Verification items for the finished model (mm, model axes). A direction names the side the tool comes from. Give positions to 0.01 mm unless a question says otherwise; leave off trailing zeros. Write each loop counter-clockwise with the first axis right and the second up, starting at its lowest first coordinate (ties: lowest second). Pieces come first, ordered by that corner, then holes. Notation, with made-up numbers: (12, -14) -> (59, -14) arc R5 cw to (59, -6) -> close; hole circle Ø5 at (62, -28). An arc over 180 degrees is marked (long way). Write item = value, one per line.
from build123d import *

# Parameters (mm, degrees)
BOSS_EXTRUDE1_DEPTH          = 2.286
SKETCH2_W                    = 25.4
SKETCH2_H                    = 2.286
BOSS_EXTRUDE2_DEPTH          = 20.828
F_10_0_1935_DIAMETER_HOLE1_D = 4.9149
F_10_0_1935_DIAMETER_HOLE2_D = 4.9149
F_10_0_1935_DIAMETER_HOLE3_D = 4.9149
CUT_EXTRUDE1_DEPTH           = 50.8
FILLET1_R                    = 2.54
FILLET2_R                    = 2.54


with BuildPart() as part:
    # Sketch1 → Boss-Extrude1 (new body)
    with BuildSketch(Plane(origin=(0, 0, 0), x_dir=(1, 0, 0), z_dir=(0, 1, 0))):
        Polygon((19.05, 34.925), (-19.05, 34.925), (-19.05, 4.22504843), (-63.051024839, 14.626449943), (-71.815919826, -22.451665109), (-19.05, -34.925), (19.05, -34.925), align=None)
    extrude(amount=BOSS_EXTRUDE1_DEPTH)

    # Sketch2 → Boss-Extrude2 (add)
    with BuildSketch(Plane(origin=(0, 2.286, 0), x_dir=(1, 0, 0), z_dir=(0, 1, 0))):
        with Locations((0, -33.782)):
            Rectangle(SKETCH2_W, SKETCH2_H)
    extrude(amount=BOSS_EXTRUDE2_DEPTH)

    # #10 (0.1935) Diameter Hole1 (through all)
    with Locations(Plane(origin=(0, 2.286, 0), x_dir=(1, 0, 0), z_dir=(0, 1, 0))):
        with Locations((-12.7, -24.735), (12.7, -24.735), (-12.7, 19.715), (12.7, 19.715)):
            Hole(F_10_0_1935_DIAMETER_HOLE1_D / 2)

    # #10 (0.1935) Diameter Hole2 (through all)
    with Locations(Plane(origin=(0, 0, 32.639), x_dir=(-1, 0, 0), z_dir=(0, 0, -1))):
        with Locations((0, 14.859)):
            Hole(F_10_0_1935_DIAMETER_HOLE2_D / 2)

    # #10 (0.1935) Diameter Hole3 (through all)
    with Locations(Plane(origin=(0, 2.286, 0), x_dir=(1, 0, 0), z_dir=(0, 1, 0))):
        with Locations((-48.685323349, 4.705533941), (-36.325951665, 1.783902278), (-54.528586674, -20.013209428), (-42.169214989, -22.93484109)):
            Hole(F_10_0_1935_DIAMETER_HOLE3_D / 2)

    # Sketch10 → Cut-Extrude1 (cut)
    with BuildSketch(Plane(origin=(0, 2.286, 0), x_dir=(1, 0, 0), z_dir=(0, 1, 0))):
        with BuildLine():
            Line((-9.525, -3.741848106), (9.525, -19.04176984))
            Line((9.525, -19.04176984), (9.525, 15.062702933))
            ThreePointArc((9.525, 15.062702933), (7.06755, 19.715), (9.525, 24.367297067))
            Line((9.525, 24.367297067), (9.525, 25.4))
            Line((9.525, 25.4), (-9.525, 25.4))
            Line((-9.525, 25.4), (-9.525, 24.367297067))
            ThreePointArc((-9.525, 24.367297067), (-7.06755, 19.715), (-9.525, 15.062702933))
            Line((-9.525, 15.062702933), (-9.525, -3.741848106))
        make_face()
        with BuildLine():
            Line((-7.305850206, -23.114), (4.454648276, -23.114))
            Line((4.454648276, -23.114), (-8.982344597, -12.322139669))
            Line((-8.982344597, -12.322139669), (-14.383129392, -19.359912238))
            ThreePointArc((-14.383129392, -19.359912238), (-10.060641775, -19.759230596), (-7.305850206, -23.114))
        make_face()
        with BuildLine():
            Line((-25.627859788, -23.582547729), (-12.912609208, -7.013281383))
            Line((-12.912609208, -7.013281383), (-32.528842365, -2.37620036))
            ThreePointArc((-32.528842365, -2.37620036), (-37.621695307, -3.697479064), (-41.583876796, -0.235680925))
            Line((-41.583876796, -0.235680925), (-44.888214049, 0.545431302))
            ThreePointArc((-44.888214049, 0.545431302), (-49.981066991, -0.775847401), (-53.94324848, 2.685950737))
            Line((-53.94324848, 2.685950737), (-55.972719823, 3.165697433))
            Line((-55.972719823, 3.165697433), (-60.355167316, -15.373360093))
            Line((-60.355167316, -15.373360093), (-58.325695974, -15.853106789))
            ThreePointArc((-58.325695974, -15.853106789), (-53.232843031, -14.531828086), (-49.270661542, -17.993626224))
            Line((-49.270661542, -17.993626224), (-45.96632429, -18.774738451))
            ThreePointArc((-45.96632429, -18.774738451), (-40.873471347, -17.453459748), (-36.911289858, -20.915257887))
            Line((-36.911289858, -20.915257887), (-25.627859788, -23.582547729))
        make_face()
    extrude(amount=-CUT_EXTRUDE1_DEPTH, mode=Mode.SUBTRACT)

    # Fillet1
    # the kernel refuses this fillet: 2.54 mm, written as the material it adds along each edge
    with BuildSketch(Plane(origin=(-19.05, 0, -4.22504843), x_dir=(0, 0, -1), z_dir=(0, 1, 0))) as fillet1_piece_1:
        with BuildLine():
            CenterArc((FILLET1_R * 1.26395030924, FILLET1_R), FILLET1_R, 166.7, 103.3)
            Line((FILLET1_R * 0.290771436458, FILLET1_R * 1.23004973719), (0, 0))
            Line((0, 0), (FILLET1_R * 1.26395030924, 0))
        make_face()
    extrude(amount=2.286)
    with BuildSketch(Plane(origin=(9.525, 2.286, -24.367297067), x_dir=(-0.773382110639457, 0, 0.6339401477607004), z_dir=(0, -1, 0)), Plane(origin=(-41.583876796, 2.286, 0.235680925), x_dir=(0.4390208071072497, 0, 0.8984768950434391), z_dir=(0, -1, 0)), Plane(origin=(-36.911289858, 2.286, 20.915257887), x_dir=(-0.43902080710723695, 0, -0.8984768950434453), z_dir=(0, -1, 0))) as fillet1_piece_2:
        with BuildLine():
            CenterArc((1.21025793, 2.5302202), FILLET1_R, 219.341421459, 45.629074101)
            Line((-0.754132631, 0.920012225), (0, 0))
            ThreePointArc((0, 0), (0.493789689, 0.021686706), (0.987579378, 0))
        make_face()
    extrude(amount=2.286)
    with BuildSketch(Plane(origin=(9.525, 2.286, -15.062702933), x_dir=(0, 0, 1), z_dir=(0, -1, 0)), Plane(origin=(-9.525, 2.286, -24.367297067), x_dir=(0, 0, -1), z_dir=(0, -1, 0)), Plane(origin=(-32.528842365, 2.286, 2.37620036), x_dir=(0.9731788727770777, 0, 0.23004973718814892), z_dir=(0, -1, 0)), Plane(origin=(-45.96632429, 2.286, 18.774738451), x_dir=(-0.9731788727770783, 0, -0.23004973718814611), z_dir=(0, -1, 0)), Plane(origin=(-44.888214049, 2.286, -0.545431302), x_dir=(0.9731788727770778, 0, 0.2300497371881489), z_dir=(0, -1, 0))) as fillet1_piece_3:
        with BuildLine():
            CenterArc((1.189595948, 2.54), FILLET1_R, 224.370925899, 45.629074101)
            ThreePointArc((-0.626066217, 0.763776224), (-0.296260998, 0.395636185), (0, 0))
            Line((0, 0), (1.189595948, 0))
        make_face()
    extrude(amount=2.286)
    with BuildSketch(Plane(origin=(9.525, 2.286, 19.04176984), x_dir=(-0.7796710587119345, 0, -0.6261893006168431), z_dir=(0, -1, 0))) as fillet1_piece_4:
        with BuildLine():
            CenterArc((FILLET1_R * 2.08573767417, FILLET1_R), FILLET1_R, 141.230467708, 128.769532292)
            Line((FILLET1_R * 1.30606661546, FILLET1_R * 1.62618930062), (0, 0))
            Line((0, 0), (FILLET1_R * 2.08573767417, 0))
        make_face()
    extrude(amount=2.286)
    with BuildSketch(Plane(origin=(-9.525, 2.286, 3.741848106), x_dir=(0, 0, -1), z_dir=(0, -1, 0))) as fillet1_piece_5:
        with BuildLine():
            CenterArc((FILLET1_R * 0.47944667845, FILLET1_R), FILLET1_R, 218.769532292, 51.230467708)
            Line((-FILLET1_R * 0.300224380262, FILLET1_R * 0.373810699383), (0, 0))
            Line((0, 0), (FILLET1_R * 0.47944667845, 0))
        make_face()
    extrude(amount=2.286)
    with BuildSketch(Plane(origin=(-9.525, 2.286, -15.062702933), x_dir=(0, 0, 1), z_dir=(0, -1, 0)), Plane(origin=(-49.270661542, 2.286, 17.993626224), x_dir=(0.9731788727770844, 0, 0.23004973718812088), z_dir=(0, -1, 0))) as fillet1_piece_6:
        with BuildLine():
            CenterArc((1.189595948, -2.54), FILLET1_R, 90, 45.629074101)
            ThreePointArc((-0.626066217, -0.763776224), (-0.296260998, -0.395636185), (0, 0))
            Line((0, 0), (1.189595948, 0))
        make_face()
    extrude(amount=2.286)
    with BuildSketch(Plane(origin=(-9.525, 2.286, -25.4), x_dir=(1, 0, 0), z_dir=(0, -1, 0)), Plane(origin=(9.525, 2.286, -25.4), x_dir=(0, 0, 1), z_dir=(0, -1, 0))) as fillet1_piece_7:
        with BuildLine():
            CenterArc((FILLET1_R, FILLET1_R), FILLET1_R, 180, 90)
            Line((0, FILLET1_R), (0, 0))
            Line((0, 0), (FILLET1_R, 0))
        make_face()
    extrude(amount=2.286)
    with BuildSketch(Plane(origin=(-7.305850206, 2.286, 23.114), x_dir=(1, 0, 0), z_dir=(0, -1, 0))) as fillet1_piece_8:
        with BuildLine():
            CenterArc((1.639698228, -2.54), FILLET1_R, 90, 59.392795524)
            ThreePointArc((-0.546423923, -1.246759907), (-0.235408974, -0.639948065), (0, 0))
            Line((0, 0), (1.639698228, 0))
        make_face()
    extrude(amount=2.286)
    with BuildSketch(Plane(origin=(-14.383129392, 2.286, 19.359912238), x_dir=(0.6087977522043749, 0, -0.7933254672017661), z_dir=(0, -1, 0))) as fillet1_piece_9:
        with BuildLine():
            CenterArc((4.66706616, 2.54), FILLET1_R, 165.34503033, 104.65496967)
            ThreePointArc((2.209700261, 3.182614066), (1.387122014, 1.395324661), (0, 0))
            Line((0, 0), (4.66706616, 0))
        make_face()
    extrude(amount=2.286)
    with BuildSketch(Plane(origin=(-8.982344597, 2.286, 12.322139669), x_dir=(0.7796710587119348, 0, 0.6261893006168427), z_dir=(0, -1, 0))) as fillet1_piece_10:
        with BuildLine():
            CenterArc((FILLET1_R * 1.02235985184, FILLET1_R), FILLET1_R, 178.733091006, 91.266908994)
            Line((FILLET1_R * 0.0226043062578, FILLET1_R * 1.02210993147), (0, 0))
            Line((0, 0), (FILLET1_R * 1.02235985184, 0))
        make_face()
    extrude(amount=2.286)
    with BuildSketch(Plane(origin=(4.454648276, 2.286, 23.114), x_dir=(-1, 0, 0), z_dir=(0, -1, 0))) as fillet1_piece_11:
        with BuildLine():
            CenterArc((FILLET1_R * 2.84206558138, FILLET1_R), FILLET1_R, 128.769532292, 141.230467708)
            Line((FILLET1_R * 2.21587628076, FILLET1_R * 1.77967105871), (0, 0))
            Line((0, 0), (FILLET1_R * 2.84206558138, 0))
        make_face()
    extrude(amount=2.286)
    with BuildSketch(Plane(origin=(-12.912609208, 2.286, 7.013281383), x_dir=(-0.6087977522043783, 0, 0.7933254672017636), z_dir=(0, -1, 0))) as fillet1_piece_12:
        with BuildLine():
            CenterArc((FILLET1_R * 1.54584224651, FILLET1_R), FILLET1_R, 155.797376702, 114.202623298)
            Line((FILLET1_R * 0.633740899703, FILLET1_R * 1.40996479501), (0, 0))
            Line((0, 0), (FILLET1_R * 1.54584224651, 0))
        make_face()
    extrude(amount=2.286)
    with BuildSketch(Plane(origin=(-25.627859788, 2.286, 23.582547729), x_dir=(-0.9731788727770897, 0, -0.2300497371880981), z_dir=(0, -1, 0))) as fillet1_piece_13:
        with BuildLine():
            CenterArc((FILLET1_R * 0.646896539576, FILLET1_R), FILLET1_R, 204.202623298, 65.797376702)
            Line((-FILLET1_R * 0.265204807237, FILLET1_R * 0.590035204995), (0, 0))
            Line((0, 0), (FILLET1_R * 0.646896539576, 0))
        make_face()
    extrude(amount=2.286)
    # the kernel refuses this fillet: 2.54 mm, written as the material it takes off along each edge
    with BuildSketch(Plane(origin=(-63.051024839, -6.35, -14.626449943), x_dir=(-0.23004973718809857, 0, 0.9731788727770896), z_dir=(0, 1, 0)), Plane(origin=(19.05, -6.35, -34.925), x_dir=(-1, 0, 0), z_dir=(0, 1, 0)), Plane(origin=(19.05, -6.35, 34.925), x_dir=(0, 0, -1), z_dir=(0, 1, 0)), Plane(origin=(-71.815919826, -6.35, 22.451665109), x_dir=(0.9731788727770898, 0, 0.23004973718809796), z_dir=(0, 1, 0))) as fillet1_2_piece_1:
        with BuildLine():
            CenterArc((FILLET1_R, FILLET1_R), FILLET1_R, 180, 90)
            Line((0, FILLET1_R), (0, 0))
            Line((0, 0), (FILLET1_R, 0))
        make_face()
    extrude(amount=14.986, mode=Mode.SUBTRACT)
    with BuildSketch(Plane(origin=(-19.05, -6.35, -34.925), x_dir=(1, 0, 0), z_dir=(0, 1, 0))) as fillet1_2_piece_2:
        with BuildLine():
            CenterArc((FILLET1_R, -FILLET1_R), FILLET1_R, 90, 90)
            Line((0, -FILLET1_R), (0, 0))
            Line((0, 0), (FILLET1_R, 0))
        make_face()
    extrude(amount=14.986, mode=Mode.SUBTRACT)
    with BuildSketch(Plane(origin=(-19.05, -0.740336242, 34.925), x_dir=(1, 0, 0), z_dir=(0, 1, 0))) as fillet1_2_piece_3:
        with BuildLine():
            CenterArc((FILLET1_R * 0.116588384541, FILLET1_R), FILLET1_R, 256.7, 13.3)
            Line((-FILLET1_R * 0.113461352647, FILLET1_R * 0.0268211272229), (0, 0))
            Line((0, 0), (FILLET1_R * 0.116588384541, 0))
        make_face()
    extrude(amount=3.766672484, mode=Mode.SUBTRACT)

    # Fillet2
    fillet2_edges = [part.edges().sort_by_distance(p)[0] for p in [
        (12.7, 2.286, 33.782),
        (0, 2.286, 32.639),
        (-12.7, 2.286, 33.782),
        (12.7, 23.114, 33.782),
        (-12.7, 23.114, 33.782),
    ]]
    fillet(fillet2_edges, radius=FILLET2_R)


solid = part.part
Item 1: Sectioned sample at C-C on y = 9.5. Record the cut outline in (x, z) (3 decimals).
Response values:
outline = (-12.7, 32.639) -> (12.7, 32.639) -> (12.7, 34.925) -> (-12.7, 34.925) -> close
Item 2: Go/stop test with flat-tipped pins: P1, Ø2.5, axis at y = 11.5, z = 33.5, coming from the -X side; P2, Ø8, axis at x = -12.7, z = -19.715, coming from the -Y side; P3, Ø1.8, axis at y = 1.5, z = -7, coming from the -X side; P4, Ø4.5, axis at x = 0, y = 14.859, coming from the -Z side. Record where each tip stops, or that it passes through.
Response values:
P1 = -12.7
P2 = 0
P3 = -65.07
P4 = through
Item 3: Mould release check, pull along Z, two halves, no side actions. Record for faces 1 (the cylindrical face through (-7.068, 1.159, -19.778)), 2 (the flat face through (0, 12, 32.639)), 3 (the cylindrical face through (-9.332, 1.159, -14.845)), 4 (the cylindrical face through (-11.976, 22.35, 33.766)): +Z half, -Z half, draft (parallel to the pull), parting line (faces both ways), or undercut.
Response values:
face_1 = undercut
face_2 = -Z half
face_3 = undercut
face_4 = draft
Item 4: Set-up check for faces 5 (the flat face through (-1, 11, 34.925)), 6 (the flat face through (-23.95, 1.159, 4.404)), 7 (the flat face through (12.7, 13, 34)): record each of +Z, -Z, +X, -X, +Y, -Y from which the full face is reachable in a straight line by a thin tool's end or side.
Response values:
face_5 = +Z, +X, -X, +Y, -Y
face_6 = +Y, -Y
face_7 = +Z, -Z, +X, +Y
Item 5: Sectioned sample at A-A on z = -8.5. Record the cut outline in (x, y) (3 decimals).
Response values:
outline = (-64.499, 0) -> (-37.134, 0) -> (-37.134, 2.286) -> (-64.499, 2.286) -> close; (-19.05, 0) -> (-9.525, 0) -> (-9.525, 2.286) -> (-19.05, 2.286) -> close; (9.525, 0) -> (19.05, 0) -> (19.05, 2.286) -> (9.525, 2.286) -> close
Item 6: Material ranges on line 1 (Z direction, x = 12.7, y = 1) (3 decimals); line 2 (X direction, y = 1.5, z = -2) (3 decimals); line 3 (Z direction, x = 10, y = 7.25) (3 decimals), recorded low to high.
Response values:
line_1 = -34.925 to -22.172, -17.258 to 22.278, 27.192 to 34.925
line_2 = -66.036 to -56.248, -53.625 to -38.774, -33.878 to -9.525, 9.525 to 19.05
line_3 = 32.639 to 34.925
Item 7: Sectioned sample at B-B on x = -28.5. Record the cut outline in (y, z), then the cut area to 3 significant figures.
Response values:
outline = (0, -6.46) -> (2.29, -6.46) -> (2.29, 3.33) -> (0, 3.33) -> close; (0, 22.9) -> (2.29, 22.9) -> (2.29, 32.69) -> (0, 32.69) -> close
area = 44.7 mm^2
